Source: CAD feature listing. Evaluate the final solid. Frame: model axes, mm. Face numbers are marked on the shaded views. Coordinates: 2 decimals unless noted, no trailing zeros. Order: outer loops, then holes, each group sorted by start corner. A loop starts at its lowest first (then second) coordinate and runs counter-clockwise, first axis right, second up.
```python
from build123d import *

# Parameters (mm, degrees)
SKETCH1_R           = 15
BOSS_EXTRUDE1_DEPTH = 11.425
SKETCH2_R           = 2.1
CUT_EXTRUDE1_DEPTH  = 32.178879069


with BuildPart() as part:
    # Sketch1 → Boss-Extrude1 (new, symmetric)
    with BuildSketch(Plane.XY):
        with Locations(Location((0, 0, 0), (0, 0, 180))):
            Circle(SKETCH1_R)
    extrude(amount=BOSS_EXTRUDE1_DEPTH, both=True)

    # Sketch2 → Cut-Extrude1 (cut, through all)
    with BuildSketch(Plane.XY.offset(11.425)):
        with Locations((-8, 8)):
            Circle(SKETCH2_R)
        with Locations((8, 8)):
            Circle(SKETCH2_R)
        with Locations((8, -8)):
            Circle(SKETCH2_R)
        with Locations((-8, -8)):
            Circle(SKETCH2_R)
    extrude(amount=-CUT_EXTRUDE1_DEPTH, mode=Mode.SUBTRACT)


solid = part.part
```
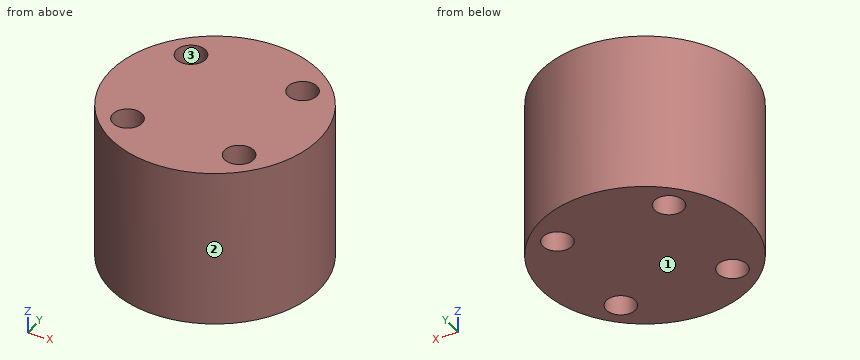
1. Section query B-B on z = -2.5. Return loops of the section in (x, y).
Findings:
outline: circle Ø30 at (0, 0); hole circle Ø4.2 at (-8, -8); hole circle Ø4.2 at (-8, 8); hole circle Ø4.2 at (8, -8); hole circle Ø4.2 at (8, 8)
2. Section query A-A on x = -7. Return loops of the section in (y, z) (1 decimal).
Findings:
outline: (-13.3, -11.4) - (-9.8, -11.4) - (-9.8, 11.4) - (-13.3, 11.4) - close; (-6.2, -11.4) - (6.2, -11.4) - (6.2, 11.4) - (-6.2, 11.4) - close; (9.8, -11.4) - (13.3, -11.4) - (13.3, 11.4) - (9.8, 11.4) - close
3. Draft query along Y for the marked faces 1, 2 and 3. Return one class per face: released by +Y, released by -Y, zero draft, split by the parting line, or undercut.
Findings:
face 1: zero draft
face 2: split by the parting line
face 3: undercut
4. Section query D-D on x = 12.75. Return loops of the section in (y, z) (3 decimals), plus the area to 3 significant figures.
Findings:
outline: (-7.902, -11.425) - (7.902, -11.425) - (7.902, 11.425) - (-7.902, 11.425) - close
area: 361 mm2
5. Ray query, line 1 (Y direction, x = -8, z = 6.25); line 2 (X direction, y = 9, z = 5.25); line 3 (Y direction, x = 9.25, z = 8.5). Return the intervals inside material, ascending.
Findings:
line 1: y = -12.69 to -10.1, -5.9 to 5.9, 10.1 to 12.69
line 2: x = -12 to -9.85, -6.15 to 6.15, 9.85 to 12
line 3: y = -11.81 to -9.69, -6.31 to 6.31, 9.69 to 11.81
6. Pin query (flat end, axial travel): P1, Ø4, axis at x = 8, y = -8, coming from the +Z side; P2, Ø8, axis at y = -8, z = 5, coming from the +X side; P3, Ø5.5, axis at x = -8, y = -8, coming from the -Z side (3 decimals); P4, Ø4, axis at y = -5.5, z = 7.5, coming from the -X side. Return the tip coordinate at first contact, or that it passes through.
Findings:
P1: passes through
P2: stops at x = 14.46
P3: stops at z = -11.425
P4: stops at x = -14.59
7. Section query C-C on y = -8. Return loops of the section in (x, z) (3 decimals).
Findings:
outline: (-12.689, -11.425) - (-10.1, -11.425) - (-10.1, 11.425) - (-12.689, 11.425) - close; (-5.9, -11.425) - (5.9, -11.425) - (5.9, 11.425) - (-5.9, 11.425) - close; (10.1, -11.425) - (12.689, -11.425) - (12.689, 11.425) - (10.1, 11.425) - close
